```python
from build123d import *

# Parameters (mm, degrees)
SKETCH1_R           = 1.4732
BOSS_EXTRUDE1_DEPTH = 3.175
FILLET1_R           = 3
FILLET2_R           = 1


with BuildPart() as part:
    # Sketch1 → Boss-Extrude1 (new body)
    with BuildSketch(Plane.XY):
        with BuildLine():
            Line((37.5, -12.587486719), (37.5, -48.86403611))
            ThreePointArc((37.5, -48.86403611), (41.119931518, -45.859516536), (44.5, -42.587486719))
            Line((44.5, -42.587486719), (44.5, -41.365734914))
            Line((44.5, -41.365734914), (44.5, -15.587486719))
            Line((44.5, -15.587486719), (44.5, -12.587486719))
            Line((44.5, -12.587486719), (37.5, -12.587486719))
        make_face()
        with Locations((40.81189221, -16.354311186)):
            Circle(SKETCH1_R, mode=Mode.SUBTRACT)
        with Locations((40.81189221, -35.404311186)):
            Circle(SKETCH1_R, mode=Mode.SUBTRACT)
    extrude(amount=BOSS_EXTRUDE1_DEPTH)

    # Fillet1
    fillet1_edges = [part.edges().sort_by_distance(p)[0] for p in [
        (44.5, -12.587486719, 1.5875),
        (44.5, -42.587486719, 1.5875),
        (37.5, -12.587486719, 1.5875),
    ]]
    fillet(fillet1_edges, radius=FILLET1_R)

    # Fillet2
    fillet2_edges = [part.edges().sort_by_distance(p)[0] for p in [
        (37.5, -48.86403611, 1.5875),
    ]]
    fillet(fillet2_edges, radius=FILLET2_R)


solid = part.part
```
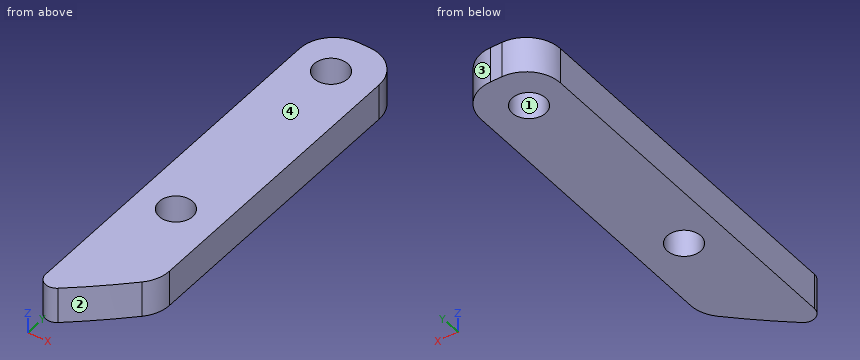
Check sheet for the modelled part. Datum: model origin and axes. Units: mm. Face numbers are marked on the shaded views. Give positions to 0.01 mm unless a question says otherwise; leave off trailing zeros. Loops run counter-clockwise (first coordinate to the right, second up) from the corner with the lowest first, then second, coordinate; pieces in that order, holes last. Notation, with made-up numbers: (54.25, 60) - (102.25, 60) arc R15 cw to (102.25, 83) - close; hole circle Ø7 at (22.25, 67.5). An arc over 180 degrees is marked (long way). One line per question, with ' | ' between items. Start each with the question number.
1. Material ranges on line 1 along X through (y, z) = (-16, 3); line 2 along Y through (x, z) = (39.5, 2.1); line 3 along Y through (x, z) = (40, 2.2), recorded low to high. Write a range as [from, to].
2. Cross-section at A-A, the plane z = 1.4. Enter the section's corners in (x, y) (3 decimals), plus the area to 3 significant figures.
3. Draft check along Y on the marked faces 1, 2, 3 and 4. Enter one of: released by +Y, released by -Y, zero draft, split by the parting line, or undercut.
4. Cross-section at B-B, the plane x = 38.75. Enter the section's corners in (y, z) (3 decimals), plus the area to 3 significant figures.
Check result:
1) line 1: x = [37.5, 39.38], [42.24, 44.5] | line 2: y = [-47.26, -36.07], [-34.73, -17.02], [-15.68, -12.76] | line 3: y = [-46.84, -36.63], [-34.18, -17.58], [-15.13, -12.63]
2) outline: (37.5, -46.792) arc R1 ccw to (39.135, -47.564) arc R61.595 ccw to (43.625, -43.484) arc R3 ccw to (44.5, -41.366) - (44.5, -15.587) arc R3 ccw to (41.5, -12.587) - (40.5, -12.587) arc R3 ccw to (37.5, -15.587) - close; hole circle Ø2.946 at (40.812, -35.404); hole circle Ø2.946 at (40.812, -16.354) | area: 214 mm2
3) face 1: undercut | face 2: released by -Y | face 3: released by +Y | face 4: zero draft
4) outline: (-47.76, 0) - (-13.151, 0) - (-13.151, 3.175) - (-47.76, 3.175) - close | area: 110 mm2
